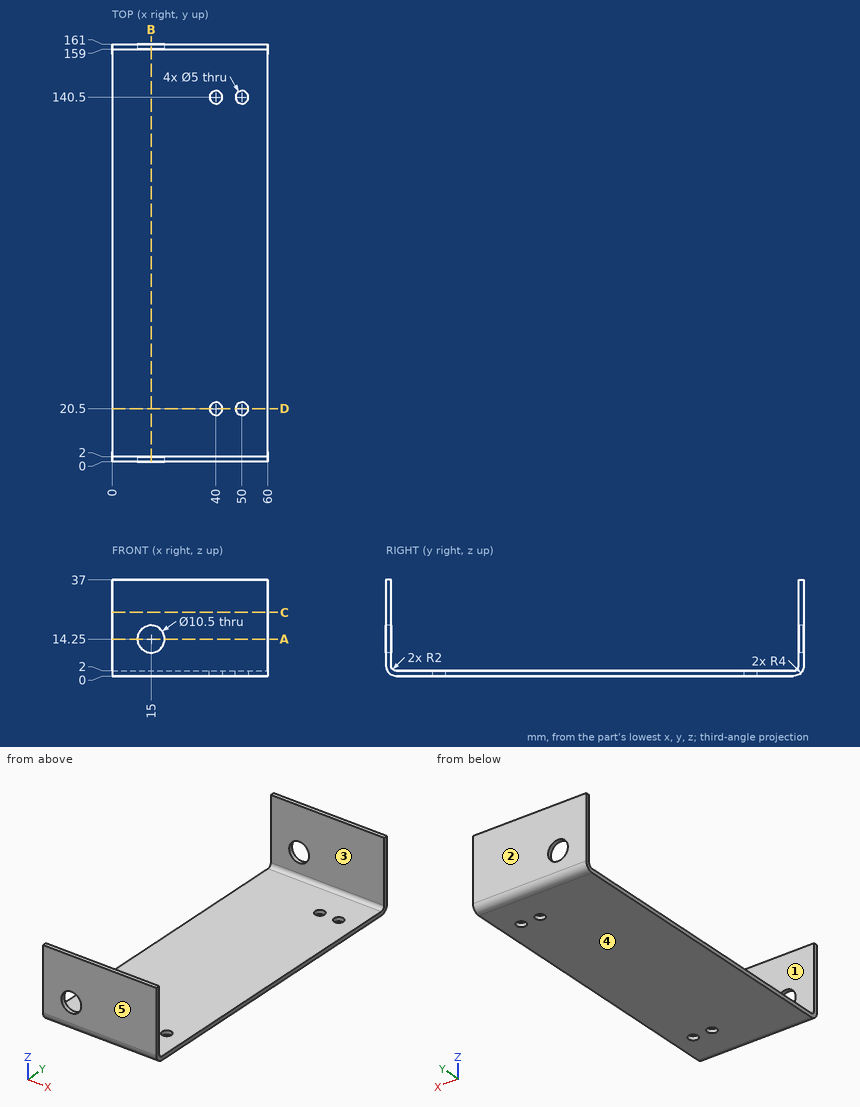
Geometry check sheet. Reference: drawing and pictorial views, mm from the part's lowest x, y, z. A direction names the side the tool comes from. Round coordinates to 2 decimals unless told otherwise and drop trailing zeros. Loops run counter-clockwise (first coordinate to the right, second up) from the corner with the lowest first, then second, coordinate; pieces in that order, holes last. Notation, with made-up numbers: (-27.75, 51.25) - (5.25, 51.25) arc R18 ccw to (5.25, 76.25) - close; hole circle Ø8 at (19, -11). An arc over 180 degrees is marked (long way). Use a Markdown table: item, result.
Q1. Cross-section at B-B on x = 15. Record the cut outline in (y, z).
Solutions:
| item | result |
|---|---|
| outline | (0, 4) arc R4 ccw to (4, 0) - (157, 0) arc R4 ccw to (161, 4) - (161, 9) - (159, 9) - (159, 4) arc R2 cw to (157, 2) - (4, 2) arc R2 cw to (2, 4) - (2, 9) - (0, 9) - close; (0, 19.5) - (2, 19.5) - (2, 37) - (0, 37) - close; (159, 19.5) - (161, 19.5) - (161, 37) - (159, 37) - close |
Q2. Go/stop test with flat-tipped pins: P1, Ø3, axis at x = 40, y = 140.5, coming from the -Z side; P2, Ø1, axis at x = 15.5, y = 90.5, coming from the +Z side. Record where each tip stops, or that it passes through.
Solutions:
| item | result |
|---|---|
| P1 | passes through |
| P2 | stops at z = 2 |
Q3. Access from +Z, -Z, +X, -X, +Y, -Y to the whole of each face (thin tool, end or side, straight path). Record for the marked faces 1 and 2.
Solutions:
| item | result |
|---|---|
| face 1 | +Z, +X, -X |
| face 2 | +Z, -Z, +X, -X, +Y |
Q4. Cross-section at D-D on y = 20.5. Record the cut outline in (x, z).
Solutions:
| item | result |
|---|---|
| outline | (0, 0) - (37.5, 0) - (37.5, 2) - (0, 2) - close; (42.5, 0) - (47.5, 0) - (47.5, 2) - (42.5, 2) - close; (52.5, 0) - (60, 0) - (60, 2) - (52.5, 2) - close |
Q5. Cross-section at C-C on z = 24.5. Record the cut outline in (x, y), plus the area to 3 significant figures.
Solutions:
| item | result |
|---|---|
| outline | (0, 0) - (60, 0) - (60, 2) - (0, 2) - close; (0, 159) - (60, 159) - (60, 161) - (0, 161) - close |
| area | 240 mm2 |
Q6. Cross-section at A-A on z = 14.25. Record the cut outline in (x, y).
Solutions:
| item | result |
|---|---|
| outline | (0, 0) - (9.75, 0) - (9.75, 2) - (0, 2) - close; (0, 159) - (9.75, 159) - (9.75, 161) - (0, 161) - close; (20.25, 0) - (60, 0) - (60, 2) - (20.25, 2) - close; (20.25, 159) - (60, 159) - (60, 161) - (20.25, 161) - close |
Q7. Draft check along Y on the marked faces 3, 4 and 5. Enter one of: released by +Y, released by -Y, zero draft, split by the parting line, or undercut.
Solutions:
| item | result |
|---|---|
| face 3 | undercut |
| face 4 | zero draft |
| face 5 | released by -Y |
Q8. Material ranges on line 1 (Y direction, x = 25, z = 4); line 2 (X direction, y = 140.5, z = 1.5); line 3 (X direction, y = 20, z = 1), recorded low to high.
Solutions:
| item | result |
|---|---|
| line 1 | y = 0 to 2, 159 to 161 |
| line 2 | x = 0 to 37.5, 42.5 to 47.5, 52.5 to 60 |
| line 3 | x = 0 to 37.55, 42.45 to 47.55, 52.45 to 60 |
